Verification items for the finished model (mm, model axes). Give positions to 0.01 mm unless a question says otherwise; leave off trailing zeros. Order: outer loops, then holes, each group sorted by start corner. A loop starts at its lowest first (then second) coordinate and runs counter-clockwise, first axis right, second up. Notation, with made-up numbers: (-31, 35.5) -> (8, 35.5) arc R17 ccw to (8, 51.5) -> close; hole circle Ø7 at (68, 11). An arc over 180 degrees is marked (long way). One line per question, with ' | ' between items. Start each with the question number.
Q1. Material ranges on probe 1 along Z at (x, y) = (-3, -0.5); probe 2 along Y at (x, z) = (17, 22); probe 3 along Y at (x, z) = (-7, 7.5), recorded low to high. Write a range as [from, to].
Q2. Go/stop test with flat-tipped pins: pin 1 (4 mm diameter, centred on x = 3.5, y = 9.5, fed in from -Z); pin 2 (6 mm diameter, centred on x = -5.5, z = -9, fed in from -Y); pin 3 (1.5 mm diameter, centred on x = -9, z = -21.5, fed in from -Y). Record where each tip stops, or that it passes through.
Q3. Section check B-B on x = -9.5. Record the cut outline in (y, z).
Q4. Section check C-C on y = 11. Record the cut outline in (x, z).
Q5. Section check D-D on x = 1. Record the cut outline in (y, z), plus the area to 3 significant figures.
Q6. Section check A-A on z = -18. Record the cut outline in (x, y), plus the area to 3 significant figures.
from build123d import *

# Parameters (mm, degrees)
F1_DEPTH = 30.48
F2_DEPTH = 25.4


with BuildPart() as f1:
    # F0 (on Top) → F1 (new body)
    with BuildSketch(Plane.XY):
        Polygon((-16.620932, 9.818526), (-17.898666, 7.23164), (-18.776572, 4.483211), (-19.235041, 1.634634), (-19.263831, -1.250458), (-19.250389, -1.346106), (-19.235041, 0.191944), (0, 0), (0.192627, 19.303413), (-2.686549, 19.116519), (-5.505712, 18.502594), (-8.201886, 17.475351), (-10.714844, 16.057738), (-12.98845, 14.281422), (-14.971915, 12.186083), align=None)
    extrude(amount=-F1_DEPTH)

    # F0 (on Top) → F2 (join)
    with BuildSketch(Plane.XY):
        Polygon((-16.620932, 9.818526), (-17.898666, 7.23164), (-18.776572, 4.483211), (-19.235041, 1.634634), (-19.263831, -1.250458), (-19.250389, -1.346106), (-19.235041, 0.191944), (0, 0), (0.192627, 19.303413), (-2.686549, 19.116519), (-5.505712, 18.502594), (-8.201886, 17.475351), (-10.714844, 16.057738), (-12.98845, 14.281422), (-14.971915, 12.186083), align=None)
        Polygon((-19.235041, 0.191944), (-19.250389, -1.346106), (-18.874113, -4.023554), (-18.039414, -6.873017), (-16.813559, -9.484887), (-15.212117, -11.884879), (-13.27086, -14.019383), (-11.033155, -15.840717), (-8.548988, -17.308196), (-5.87385, -18.389038), (-3.0675, -19.0591), (-0.192627, -19.303413), (0, 0), align=None)
        Polygon((-18.874113, -4.023554), (-19.250389, -1.346106), (-19.263831, -2.693147), align=None)
        Polygon((-18.039414, -6.873017), (-18.874113, -4.023554), (-18.862299, -4.107616), align=None)
        Polygon((0.192627, 19.303413), (0, 0), (19.249436, -0.192088), (19.263831, 1.250458), (18.862299, 4.107616), (18.039414, 6.873017), (16.813559, 9.484887), (15.212117, 11.884879), (13.27086, 14.019383), (11.033155, 15.840717), (8.548988, 17.308196), (5.87385, 18.389038), (3.0675, 19.0591), align=None)
        Polygon((19.249436, -0.192088), (0, 0), (-0.192627, -19.303413), (2.686549, -19.116519), (5.505712, -18.502594), (8.201886, -17.475351), (10.714844, -16.057738), (12.98845, -14.281422), (14.971915, -12.186083), (16.620932, -9.818526), (17.898666, -7.23164), (18.776572, -4.483211), (19.235041, -1.634634), align=None)
        Polygon((19.263831, -0.192232), (19.249436, -0.192088), (19.235041, -1.634634), align=None)
    extrude(amount=F2_DEPTH)


solid = f1.part
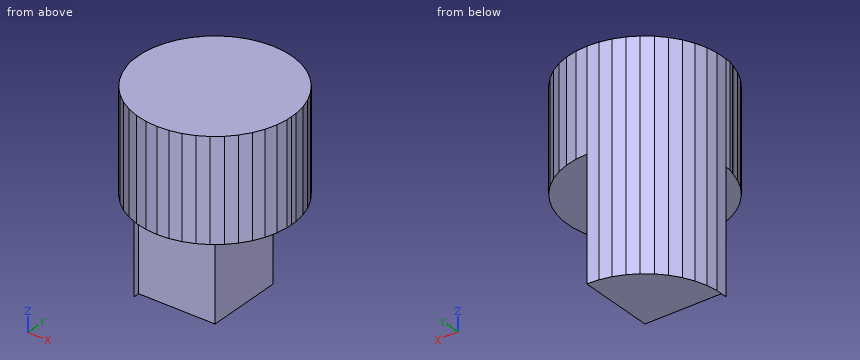
Filled in:
1) probe 1: [0, 25.4] | probe 2: [-9.05, 9.09] | probe 3: [-17.93, 17.93]
2) pin 1: z = 0 | pin 2: y = 0.02 | pin 3: y = 0.08
3) outline: (-16.75, 0) -> (0.09, 0) -> (0.09, -30.48) -> (16.74, -30.48) -> (16.74, 25.4) -> (-16.75, 25.4) -> close
4) outline: (-15.8, -30.48) -> (0.11, -30.48) -> (0.11, 0) -> (15.8, 0) -> (15.8, 25.4) -> (-15.8, 25.4) -> close
5) outline: (-19.23, 0) -> (19.23, 0) -> (19.23, 25.4) -> (-19.23, 25.4) -> close | area: 977 mm²
6) outline: (-19.26, -1.25) -> (-19.25, -1.35) -> (-19.24, 0.19) -> (0, 0) -> (0.19, 19.3) -> (-2.69, 19.12) -> (-5.51, 18.5) -> (-8.2, 17.48) -> (-10.71, 16.06) -> (-12.99, 14.28) -> (-14.97, 12.19) -> (-16.62, 9.82) -> (-17.9, 7.23) -> (-18.78, 4.48) -> (-19.24, 1.63) -> close | area: 292 mm²
